Part print with two shaded views. Sizes in mm from the minimum x, y, z corner. A direction names the side the tool comes from. Coordinates: 2 decimals unless noted, no trailing zeros. Loops run counter-clockwise (first coordinate to the right, second up) from the corner with the lowest first, then second, coordinate; pieces in that order, holes last.
Item 1: Cut at C-C (z = 23). List the corners of the cut face in (x, y), and give its area (3 significant figures).
Item 2: Cut at B-B (y = 19.5). List the corners of the cut face in (x, z), and give its area (4 significant figures).
Item 3: Cut at D-D (y = 46). List the corners of the cut face in (x, z), and give its area (3 significant figures).
Item 4: 3-axis set-ups, long thin cutter, end or side, ignore diameter. For the marked faces 1 and 2: which of +Z, -Z, +X, -X, +Y, -Y reach the whole face in a straight line?
Item 5: Cut at A-A (x = 25.4). List the corners of the cut face in (y, z), and give its area (3 significant figures).
Item 6: Drill centre lines: line 1 along Z through (x, y) = (25, 36); line 2 along X through (y, z) = (12, 50) (1 decimal); line 3 along Y through (x, z) = (60, 28.5). Where is each one in solid material? Low to high.
Item 7: Flat gauge pins, fed straight in: pin 1 (3 mm diameter, centred on y = 31, z = 68, fed in from +X); pin 2 (20.5 mm diameter, centred on y = 7.5, z = 29.5, fed in from +X); pin 3 (4 mm diameter, centred on x = 53.5, y = 18, fed in from +Z). Where does each tip first touch, or does it go through?
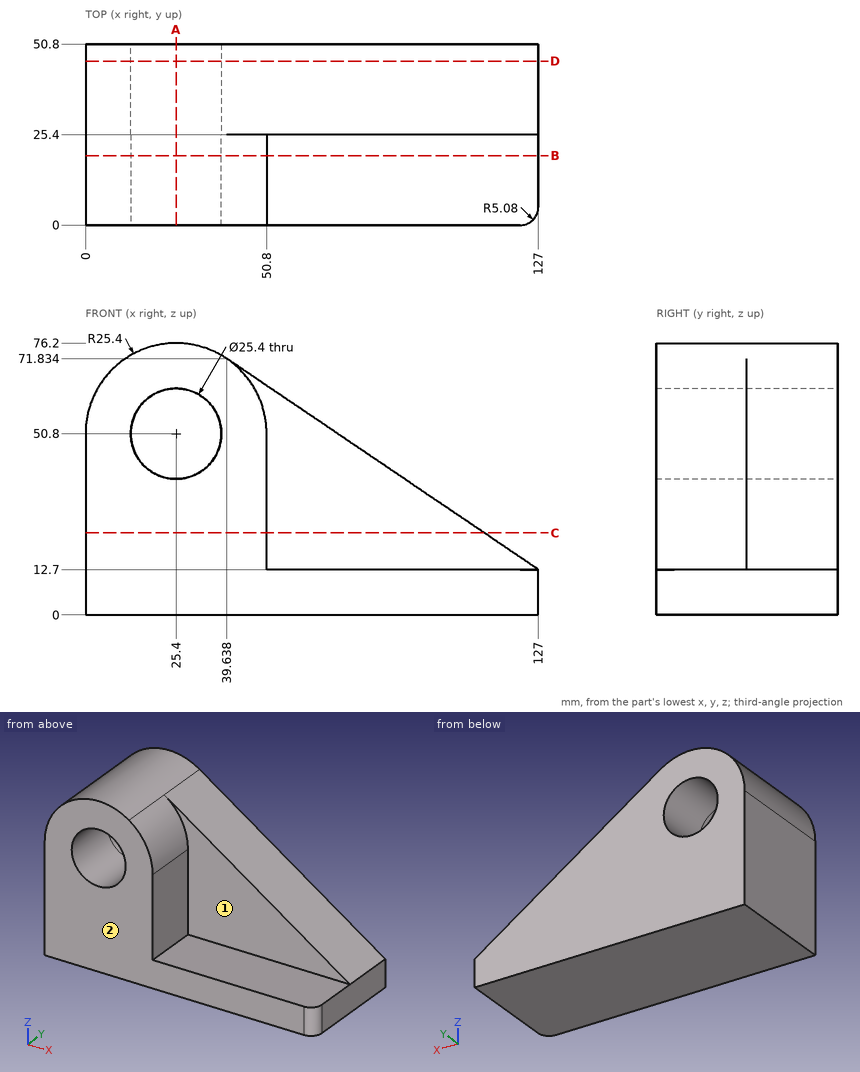
Filled sheet:
1. outline: (0, 0) - (50.8, 0) - (50.8, 25.4) - (111.78, 25.4) - (111.78, 50.8) - (0, 50.8) - close
1. area: 4,130 mm2
2. outline: (0, 0) - (127, 0) - (127, 12.7) - (50.8, 12.7) - (50.8, 50.8) arc R25.4 ccw to (0, 50.8) - close; hole circle Ø25.4 at (25.4, 50.8)
2. area: 4,055 mm2
3. outline: (0, 0) - (127, 0) - (127, 12.7) - (39.64, 71.83) arc R25.4 ccw to (0, 50.8) - close; hole circle Ø25.4 at (25.4, 50.8)
3. area: 6,050 mm2
4. face 1: +Z, +X, -Y
4. face 2: +Z, -Z, +X, -X, -Y
5. outline: (0, 0) - (50.8, 0) - (50.8, 38.1) - (0, 38.1) - close; (0, 63.5) - (50.8, 63.5) - (50.8, 76.2) - (0, 76.2) - close
5. area: 2,580 mm2
6. line 1: z = 0 to 38.11, 63.49 to 76.2
6. line 2: x = 0 to 12.7, 38.1 to 50.8
6. line 3: y = 25.4 to 50.8
7. pin 1: stops at x = 47.52
7. pin 2: stops at x = 50.8
7. pin 3: stops at z = 12.7
